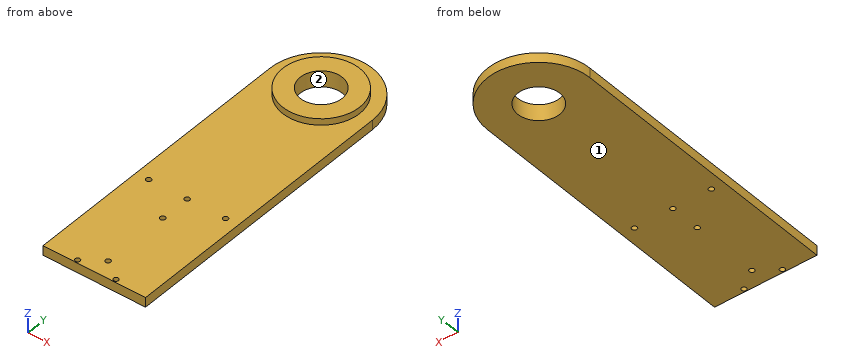
```python
from build123d import *

# Parameters (mm, degrees)
BOSS_EXTRUDE1_DEPTH              = 9.525
SKETCH2_R                        = 38.1
BOSS_EXTRUDE2_DEPTH              = 6.35
SKETCH3_R                        = 20.7645
CUT_EXTRUDE1_DEPTH               = 335.461799949
F_10_0_1935_DIAMETER_HOLE1_D     = 4.9149
F_10_0_1935_DIAMETER_HOLE1_DEPTH = 10.16
F_10_0_1935_DIAMETER_HOLE1_TIP   = 1.476584928
F_10_CLEARANCE_HOLE1_D           = 5.1054


with BuildPart() as part:
    # Sketch1 → Boss-Extrude1 (new body)
    with BuildSketch(Plane.XY):
        with BuildLine():
            Line((-50.8, 0), (50.8, 0))
            Line((50.8, 0), (50.8, 279.4))
            ThreePointArc((50.8, 279.4), (0, 330.2), (-50.8, 279.4))
            Line((-50.8, 279.4), (-50.8, 0))
        make_face()
    extrude(amount=BOSS_EXTRUDE1_DEPTH)

    # Sketch2 → Boss-Extrude2 (add)
    with BuildSketch(Plane.XY.offset(9.525)):
        with Locations((0, 279.4)):
            Circle(SKETCH2_R)
    extrude(amount=BOSS_EXTRUDE2_DEPTH)

    # Sketch3 → Cut-Extrude1 (cut, through all)
    with BuildSketch(Plane.XY.offset(15.875)):
        with Locations((0, 279.4)):
            Circle(SKETCH3_R)
    extrude(amount=-CUT_EXTRUDE1_DEPTH, mode=Mode.SUBTRACT)

    # #10 (0.1935) Diameter Hole1
    with Locations(Plane(origin=(0, 0, 0), x_dir=(-1, 0, 0), z_dir=(0, 0, -1))):
        with Locations((-19.05, 3.175), (19.05, 3.175)):
            Hole(F_10_0_1935_DIAMETER_HOLE1_D / 2, depth=F_10_0_1935_DIAMETER_HOLE1_DEPTH)
            with Locations((0, 0, -(F_10_0_1935_DIAMETER_HOLE1_DEPTH + F_10_0_1935_DIAMETER_HOLE1_TIP / 2))):  # 118° drill point
                Cone(0, F_10_0_1935_DIAMETER_HOLE1_D / 2, F_10_0_1935_DIAMETER_HOLE1_TIP, mode=Mode.SUBTRACT)

    # #10 Clearance Hole1 (through all)
    with Locations(Plane(origin=(0, 0, 0), x_dir=(-1, 0, 0), z_dir=(0, 0, -1))):
        with Locations((0, 84.30006), (0, 16.99006), (-38.1, 114.3), (0, 114.3), (38.1, 114.3)):
            Hole(F_10_CLEARANCE_HOLE1_D / 2)


solid = part.part
```
Source: CAD feature listing. Evaluate the final solid. Frame: model axes, mm. Face numbers are marked on the shaded views. Give positions to 0.01 mm unless a question says otherwise; leave off trailing zeros. Loops run counter-clockwise (first coordinate to the right, second up) from the corner with the lowest first, then second, coordinate; pieces in that order, holes last. Notation, with made-up numbers: (45, -8.75) - (66, -8.75) arc R24 cw to (66, 23.25) - close; hole circle Ø10 at (49.5, -4). An arc over 180 degrees is marked (long way). Use CSV: the item, a comma, the result in double quotes.
1) Pin query (flat end, axial travel): P1, Ø6, axis at x = -18.5, z = 11, coming from the +Y side; P2, Ø3, axis at x = 0, y = 114.3, coming from the +Z side; P3, Ø8, axis at x = 0, y = 84.3, coming from the +Z side (3 decimals). Return the tip coordinate at first contact, or that it passes through.
Worked out:
P1,"stops at y = 327.65"
P2,"passes through"
P3,"stops at z = 9.525"
2) Mould query, pull axis Y, two halves, no side actions, for the marked faces 1 and 2. Classes: +Y half, -Y half, draft (parallel to the pull), parting line (faces both ways), or undercut.
Worked out:
face 1,"draft"
face 2,"undercut"
3) Line query: line 1 (Y direction, x = 0, z = 4.75); line 2 (Y direction, x = -19.05, z = 6); line 3 (Z direction, x = 42, y = 269.5) (3 decimals). Output: solid intervals per line, ascending.
Worked out:
line 1,"y = 0 to 14.44, 19.54 to 81.75, 86.85 to 111.75, 116.85 to 258.64, 300.16 to 330.2"
line 2,"y = 0 to 0.72, 5.63 to 271.14, 287.66 to 326.49"
line 3,"z = 0 to 9.525"
4) Cut plane B-B (x = -13.5). Output: boundary loops of the cut face in (y, z) (3 decimals), and give its area (3 significant figures).
Worked out:
outline,"(0, 0) - (263.623, 0) - (263.623, 15.875) - (243.772, 15.875) - (243.772, 9.525) - (0, 9.525) - close; (295.177, 0) - (328.373, 0) - (328.373, 9.525) - (315.028, 9.525) - (315.028, 15.875) - (295.177, 15.875) - close"
area,"3,080 mm^2"
5) Cut plane C-C (x = -31). Output: boundary loops of the cut face in (y, z) (3 decimals), and give its area (3 significant figures).
Worked out:
outline,"(0, 0) - (319.645, 0) - (319.645, 9.525) - (301.55, 9.525) - (301.55, 15.875) - (257.25, 15.875) - (257.25, 9.525) - (0, 9.525) - close"
area,"3,330 mm^2"
6) Cut plane A-A (z = 5.75). Count the separate pieces of the cut face and the enclosed holes in it, and give its area (3 significant figures).
Worked out:
separate pieces,"1"
enclosed holes,"8"
area,"30,900 mm^2"
7) Cut plane D-D (y = 69.5). Output: boundary loops of the cut face in (x, z) (3 decimals).
Worked out:
outline,"(-50.8, 0) - (50.8, 0) - (50.8, 9.525) - (-50.8, 9.525) - close"
